The drawing under review shows one solid part. Ordinate dimensions are in mm from its lowest x, y, z. Coordinates: 2 decimals unless noted, no trailing zeros. Order: outer loops, then holes, each group sorted by start corner. A loop starts at its lowest first (then second) coordinate and runs counter-clockwise, first axis right, second up. Notation, with made-up numbers: (-5.5, 68.25) -> (29.5, 68.25) arc R20 ccw to (29.5, 95.25) -> close; hole circle Ø4 at (19.5, -7.5). An arc over 180 degrees is marked (long way). Write item = value, one per line.
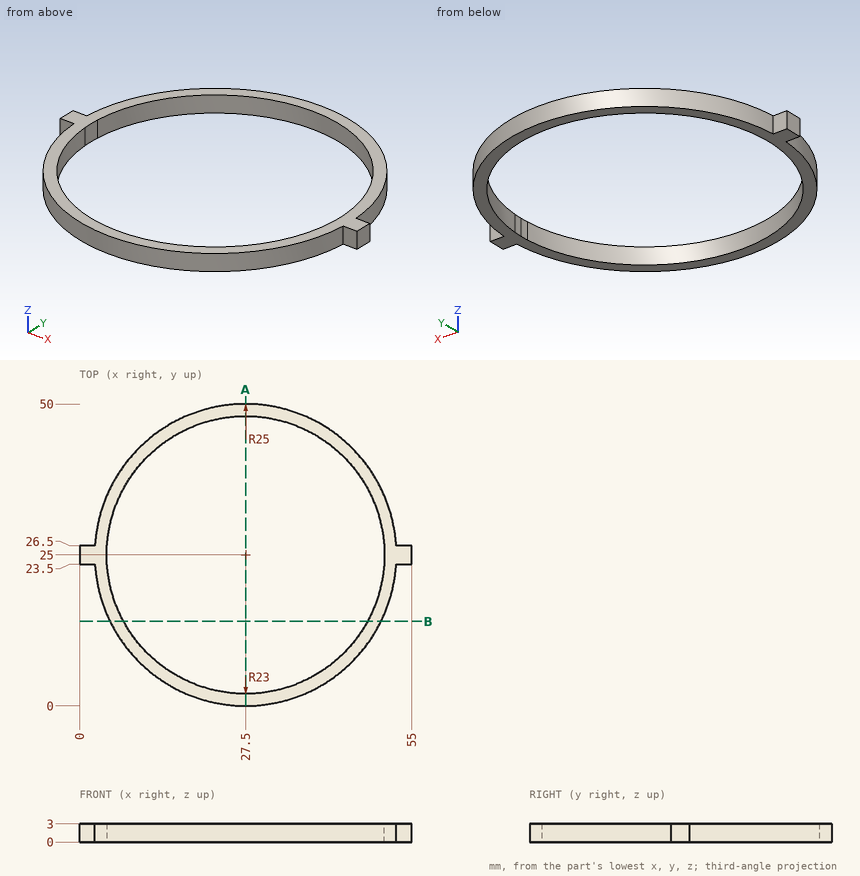
(1) For L1, parallel to Y at x = 30, z = 2.5; L2, parallel to X at y = 40.5, z = 0.9; L3, parallel to Y at x = 48, z = 2, list the stretches that pass through material, from the lowest coordinate up.
Report:
L1 = 0.13 to 2.14, 47.86 to 49.87
L2 = 7.88 to 10.51, 44.49 to 47.12
L3 = 10.69 to 14.57, 35.43 to 39.31
(2) We need section B-B (y = 14). Write out the cut boundary in (x, z).
Report:
outline = (5.05, 0) -> (7.3, 0) -> (7.3, 3) -> (5.05, 3) -> close; (47.7, 0) -> (49.95, 0) -> (49.95, 3) -> (47.7, 3) -> close
(3) We need section A-A (x = 27.5). Write out the cut boundary in (y, z).
Report:
outline = (0, 0) -> (2, 0) -> (2, 3) -> (0, 3) -> close; (48, 0) -> (50, 0) -> (50, 3) -> (48, 3) -> close
(4) Insertion check: pin 1 (5 mm diameter, centred on x = 8, y = 31.5, fed in from +Z); pin 2 (1 mm diameter, centred on y = 5, z = 1, fed in from -X); pin 3 (0.8 mm diameter, centred on x = 1.5, z = 2, fed in from -Y). Each pin has a flat end and moves straight along its axis. Give the tip position at first contact, or say it passes through.
Report:
pin_1 = 3
pin_2 = 11.86
pin_3 = 23.5
